```python
from build123d import *

# Parameters (mm, degrees)
REAR_COVER_REFERENCE_START   = -47
SKETCH_1_R                   = 78.5
SKETCH_1_R_2                 = 17.5
REAR_COVER_REFERENCE_DEPTH   = 2.5
BEARING_BOSS_REFERENCE_START = -47
SKETCH_2_R                   = 23
SKETCH_2_R_2                 = 17.5
BEARING_BOSS_REFERENCE_DEPTH = 10
SKETCH_3_R                   = 6.5
THROUGH_HOLES_DEPTH          = 100


with BuildPart() as part:
    # Эскиз1 → Rear_cover_reference (new body)
    with BuildSketch(Plane.XY.offset(REAR_COVER_REFERENCE_START)):
        Circle(SKETCH_1_R)
        Circle(SKETCH_1_R_2, mode=Mode.SUBTRACT)
    extrude(amount=REAR_COVER_REFERENCE_DEPTH)

    # Эскиз2 → Bearing_boss_reference (add)
    with BuildSketch(Plane.XY.offset(BEARING_BOSS_REFERENCE_START)):
        Circle(SKETCH_2_R)
        Circle(SKETCH_2_R_2, mode=Mode.SUBTRACT)
    extrude(amount=BEARING_BOSS_REFERENCE_DEPTH)

    # Эскиз3 → Through_holes (cut, symmetric)
    with BuildSketch(Plane.XY):
        with Locations((40, 0)):
            Circle(SKETCH_3_R)
        with Locations((34.641016151, 20)):
            Circle(SKETCH_3_R)
        with Locations((20, 34.641016151)):
            Circle(SKETCH_3_R)
        with Locations((0, 40)):
            Circle(SKETCH_3_R)
        with Locations((-20, 34.641016151)):
            Circle(SKETCH_3_R)
        with Locations((-34.641016151, 20)):
            Circle(SKETCH_3_R)
        with Locations((-40, 0)):
            Circle(SKETCH_3_R)
        with Locations((-34.641016151, -20)):
            Circle(SKETCH_3_R)
        with Locations((-20, -34.641016151)):
            Circle(SKETCH_3_R)
        with Locations((0, -40)):
            Circle(SKETCH_3_R)
        with Locations((20, -34.641016151)):
            Circle(SKETCH_3_R)
        with Locations((34.641016151, -20)):
            Circle(SKETCH_3_R)
        with Locations((62.785178709, 16.823237932)):
            Circle(SKETCH_3_R)
        with Locations((45.961940777, 45.961940777)):
            Circle(SKETCH_3_R)
        with Locations((16.823237932, 62.785178709)):
            Circle(SKETCH_3_R)
        with Locations((-16.823237932, 62.785178709)):
            Circle(SKETCH_3_R)
        with Locations((-45.961940777, 45.961940777)):
            Circle(SKETCH_3_R)
        with Locations((-62.785178709, 16.823237932)):
            Circle(SKETCH_3_R)
        with Locations((-62.785178709, -16.823237932)):
            Circle(SKETCH_3_R)
        with Locations((-45.961940777, -45.961940777)):
            Circle(SKETCH_3_R)
        with Locations((-16.823237932, -62.785178709)):
            Circle(SKETCH_3_R)
        with Locations((16.823237932, -62.785178709)):
            Circle(SKETCH_3_R)
        with Locations((45.961940777, -45.961940777)):
            Circle(SKETCH_3_R)
        with Locations((62.785178709, -16.823237932)):
            Circle(SKETCH_3_R)
    extrude(amount=THROUGH_HOLES_DEPTH, both=True, mode=Mode.SUBTRACT)


solid = part.part
```
CAD build for the part. Positions are in the model's coordinates, mm. Coordinates: 2 decimals unless noted, no trailing zeros. Order: outer loops, then holes, each group sorted by start corner. A loop starts at its lowest first (then second) coordinate and runs counter-clockwise, first axis right, second up. Notation, with made-up numbers: M -37.75,-7 L -33.75,-7 A25 ccw -33.75,19 Z; hole C 70.25,12 d1. An arc over 180 degrees is marked long. Answer as CSV lines item,"result".
1) Cut at B-B (x = 0.5). List the corners of the cut face in (y, z).
Verdict:
outline,"M -78.5,-47 L -46.48,-47 L -46.48,-44.5 L -78.5,-44.5 Z; M -33.52,-47 L -17.49,-47 L -17.49,-37 L -22.99,-37 L -22.99,-44.5 L -33.52,-44.5 Z; M 17.49,-47 L 33.52,-47 L 33.52,-44.5 L 22.99,-44.5 L 22.99,-37 L 17.49,-37 Z; M 46.48,-47 L 78.5,-47 L 78.5,-44.5 L 46.48,-44.5 Z"
2) Drill centre lines: L1, parallel to X at y = -33, z = -46; L2, parallel to X at y = -6, z = -45.75; L3, parallel to Z at x = 14, y = 39.5. Where is each one in solid material? Low to high. Write a range as from..to.
Verdict:
L1,"-71.23..-26.29, -13.71..13.71, 26.29..71.23"
L2,"-78.27..-42.5, -37.5..-16.44, 16.44..37.5, 42.5..78.27"
L3,"-47..-44.5"
3) Flat gauge pins, fed straight in: P1, Ø15, axis at x = -62.79, y = 16.82, coming from the +Z side; P2, Ø11.5, axis at x = -16.82, y = 62.79, coming from the +Z side; P3, Ø15, axis at x = 16.82, y = 62.79, coming from the -Z side; P4, Ø6, axis at y = 22.5, z = -40, coming from the +X side. Where does each tip first touch, or does it go through?
Verdict:
P1,"z = -44.5"
P2,"through"
P3,"z = -47"
P4,"x = 12.2"
4) Cut at C-C (y = -65.5). List the corners of the cut face in (x, z), then the cut area to 3 significant figures.
Verdict:
outline,"M -43.27,-47 L -22.73,-47 L -22.73,-44.5 L -43.27,-44.5 Z; M -10.92,-47 L 10.92,-47 L 10.92,-44.5 L -10.92,-44.5 Z; M 22.73,-47 L 43.27,-47 L 43.27,-44.5 L 22.73,-44.5 Z"
area,"157 mm2"
5) Mould opens along Y. For faces 1 (the cylindrical face through (-52.456, 46.248, -45.732)), 2 (the cylindrical face through (-2.994, 22.804, -40.802)), 3 (the flat face through (-19, 19, -44.5)) say: released by +Y, released by -Y, zero draft, split by the parting line, or undercut.
Verdict:
face 1,"undercut"
face 2,"split by the parting line"
face 3,"zero draft"
6) Cut at D-D (x = 60.5). List the corners of the cut face in (y, z), then the cut area to 3 significant figures.
Verdict:
outline,"M -50.02,-47 L -22.91,-47 L -22.91,-44.5 L -50.02,-44.5 Z; M -10.74,-47 L 10.74,-47 L 10.74,-44.5 L -10.74,-44.5 Z; M 22.91,-47 L 50.02,-47 L 50.02,-44.5 L 22.91,-44.5 Z"
area,"189 mm2"
7) Cut at A-A (y = 0). List the corners of the cut face in (x, z).
Verdict:
outline,"M -78.5,-47 L -46.5,-47 L -46.5,-44.5 L -78.5,-44.5 Z; M -33.5,-47 L -17.5,-47 L -17.5,-37 L -23,-37 L -23,-44.5 L -33.5,-44.5 Z; M 17.5,-47 L 33.5,-47 L 33.5,-44.5 L 23,-44.5 L 23,-37 L 17.5,-37 Z; M 46.5,-47 L 78.5,-47 L 78.5,-44.5 L 46.5,-44.5 Z"
